from build123d import *

# Parameters (mm, degrees)
BOSS_EXTRUDE1_DEPTH = 12.7
SKETCH2_W           = 44.45
SKETCH2_H           = 19.05
CUT_EXTRUDE1_DEPTH  = 60.652834174


with BuildPart() as part:
    # Sketch1 → Boss-Extrude1 (new, symmetric)
    with BuildSketch(Plane.XY):
        Polygon((19.05, -50.8), (19.05, 0), (-28.575, 0), (9.525, 44.45), (9.525, 31.75), (22.225, 31.75), (22.225, -50.8), align=None)
    extrude(amount=BOSS_EXTRUDE1_DEPTH, both=True)

    # Sketch2 → Cut-Extrude1 (cut, through all)
    with BuildSketch(Plane.XZ):
        with Locations((-3.175, 0)):
            Rectangle(SKETCH2_W, SKETCH2_H)
    extrude(amount=-CUT_EXTRUDE1_DEPTH, mode=Mode.SUBTRACT)


solid = part.part
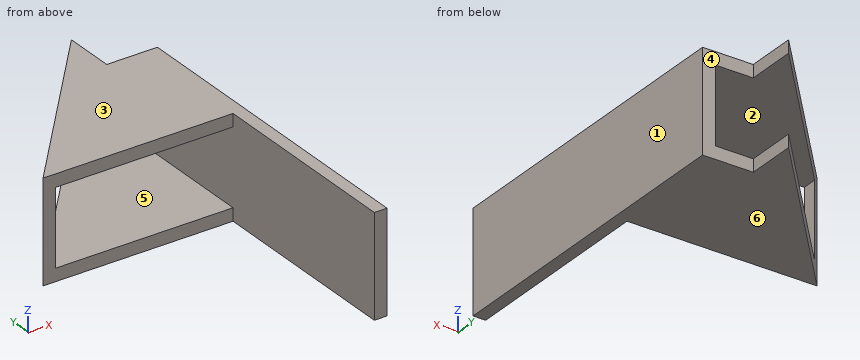
Model file for the job. Use its own axes, mm. Face numbers are marked on the shaded views. A direction names the side the tool comes from. Give positions to 0.01 mm unless a question says otherwise; leave off trailing zeros. Loops run counter-clockwise (first coordinate to the right, second up) from the corner with the lowest first, then second, coordinate; pieces in that order, holes last.
Item 1: Slice it at C-C (z = -11). Write the cut outline in (x, y) (3 decimals), plus the area to 3 significant figures.
Check values:
outline: (-28.575, 0) - (19.05, 0) - (19.05, -50.8) - (22.225, -50.8) - (22.225, 31.75) - (9.525, 31.75) - (9.525, 44.45) - close
area: 1,410 mm2
Item 2: Mould opens along Z. For the marked faces 1, 2 and 3 say: +Z half, -Z half, draft (parallel to the pull), parting line (faces both ways), or undercut.
Check values:
face 1: draft
face 2: undercut
face 3: +Z half
Item 3: Which spindle directions (+Z, -Z, +X, -X, +Y, -Y) get a long thin tool onto all of the face, cutting with end or side? Do the marked faces 4, 5 and 6. Say none if no direction does.
Check values:
face 4: +Z, -Z, +X, +Y
face 5: +Y, -Y
face 6: -Z, +X, -X, +Y, -Y
Item 4: Slice it at A-A (z = -3). Write the cut outline in (x, y) (3 decimals), plus the area to 3 significant figures.
Check values:
outline: (-28.575, 0) - (-25.4, 0) - (-25.4, 3.704) - close; (19.05, -50.8) - (22.225, -50.8) - (22.225, 31.75) - (19.05, 31.75) - close
area: 268 mm2
Item 5: Slice it at B-B (x = -6). Write the cut outline in (y, z) (1 decimal).
Check values:
outline: (0, -12.7) - (26.3, -12.7) - (26.3, -9.5) - (0, -9.5) - close; (0, 9.5) - (26.3, 9.5) - (26.3, 12.7) - (0, 12.7) - close
Item 6: Drill centre lines: line 1 along Z through (x, y) = (11, 24.5) (3 decimals); line 2 along X through (y, z) = (-35.5, 11.5) (3 decimals); line 3 along Y through (x, z) = (14, -11). Where is each one in solid material? Low to high.
Check values:
line 1: z = -12.7 to -9.525, 9.525 to 12.7
line 2: x = 19.05 to 22.225
line 3: y = 0 to 31.75
Item 7: Drop flat-ended pins along their axis: P1, Ø2, axis at x = -22.5, z = 1, coming from the +Y side; P2, Ø4, axis at x = -16.5, z = -9, coming from the -Y side; P3, Ø13.5, axis at x = -7.5, y = 33, coming from the -Z side; P4, Ø2.5, axis at y = 38, z = -10.5, coming from the +X side (3 decimals). Give the stop position or say it passes through.
Check values:
P1: passes through
P2: stops at y = 0
P3: stops at z = -12.7
P4: stops at x = 9.525
Item 8: Slice it at D-D (x = 15.5). Write the cut outline in (y, z) (3 decimals).
Check values:
outline: (0, -12.7) - (31.75, -12.7) - (31.75, -9.525) - (0, -9.525) - close; (0, 9.525) - (31.75, 9.525) - (31.75, 12.7) - (0, 12.7) - close
